Input: dimensioned drawing with shaded views. Units: mm. Origin: part minimum x, y, z. Round coordinates to 2 decimals unless told otherwise and drop trailing zeros. Loops run counter-clockwise (first coordinate to the right, second up) from the corner with the lowest first, then second, coordinate; pieces in that order, holes last.
1) Ray query, line 1 along X through (y, z) = (16, 51); line 2 along X through (y, z) = (28, 59). Return the intervals inside material, ascending.
2) First-contact query: pin 1 (2 mm diameter, centred on y = 14.5, z = 55, fed in from +X); pin 2 (8 mm diameter, centred on x = 53, y = 18.5, fed in from -Z); pin 3 (8 mm diameter, centred on x = 32.5, y = 29.5, fed in from +Z). Flat tips, straight axial feed; report the tip coordinate or a pass-through.
3) Section B-B, the plane x = 16.5. Return loops of the section in (y, z).
4) Section A-A, the plane z = 51. Return loops of the section in (x, y), and give its area (3 significant figures).
5) Draft query along Z for the marked faces 1 and 2. Return one class per face: pulls with the +Z half, pulls with the -Z half, needs draft (parallel to the pull), parting line crosses it, or undercut.
6) Section C-C, the plane y = 7.5. Return loops of the section in (x, z).
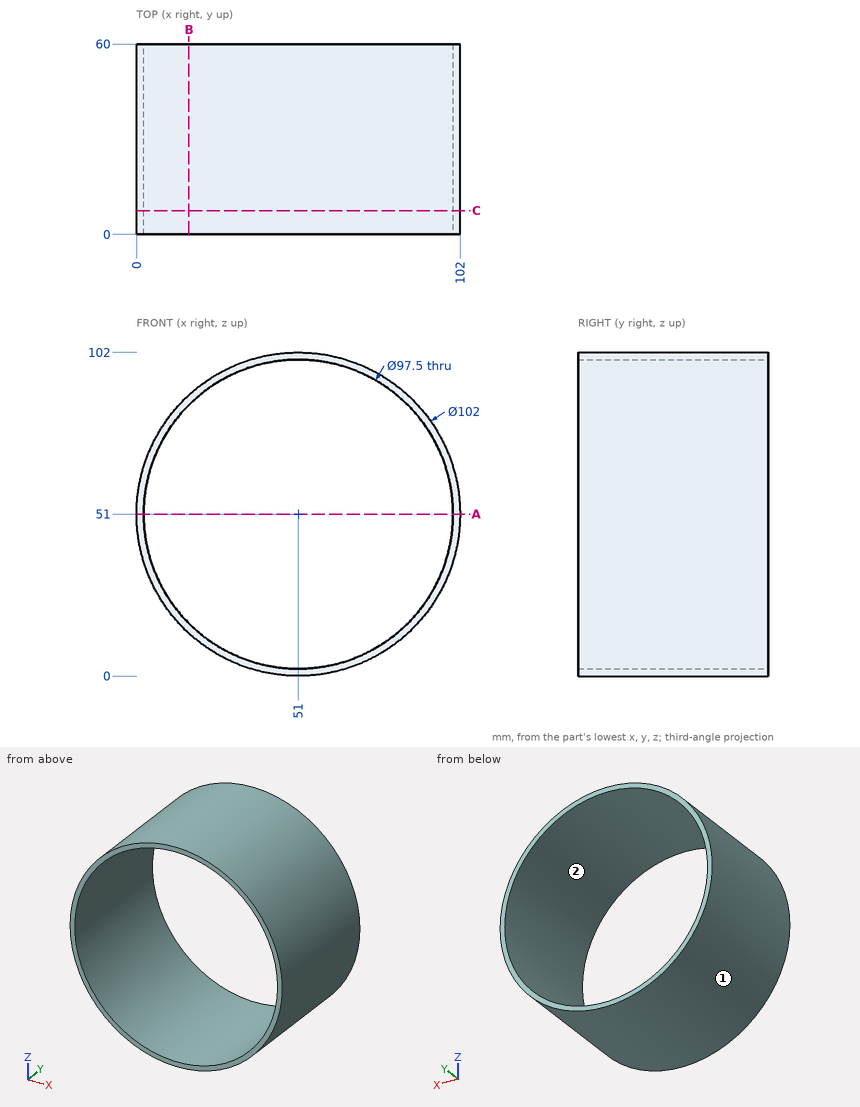
Final values:
1. line 1: x = 0 to 2.25, 99.75 to 102
1. line 2: x = 0.63 to 2.91, 99.09 to 101.37
2. pin 1: stops at x = 101.91
2. pin 2: stops at z = 0
2. pin 3: stops at z = 99.9
3. outline: (0, 13.44) - (60, 13.44) - (60, 16.56) - (0, 16.56) - close; (0, 85.44) - (60, 85.44) - (60, 88.56) - (0, 88.56) - close
4. outline: (0, 0) - (2.25, 0) - (2.25, 60) - (0, 60) - close; (99.75, 0) - (102, 0) - (102, 60) - (99.75, 60) - close
4. area: 270 mm2
5. face 1: parting line crosses it
5. face 2: undercut
6. outline: circle Ø102 at (51, 51); hole circle Ø97.5 at (51, 51)
